```python
from build123d import *

# Parameters (mm, degrees)
F1_DEPTH = 18


with BuildPart() as f1:
    # F0 (on Front) → F1 (new body)
    with BuildSketch(Plane.XZ):
        with BuildLine():
            Line((295, -217), (-317, -217))
            add(Edge.make_bspline(
                [(167, -341), (73.2052326202, -351.3030406237), (-82.9134855426, -352.2458970512), (-215.8919105735, -315.6215987583), (-316.2735343339, -258.65300402), (-317, -217)],
                knots=[0, 0, 0, 0, 0.4043982891, 0.7107448428, 1, 1, 1, 1], degree=3))
            Line((167, -341), (167, -329))
            Line((167, -329), (295, -329))
            Line((295, -329), (295, -217))
        make_face()
        with BuildLine():
            add(Edge.make_bspline(
                [(167, -93), (73.2052326202, -82.6969593763), (-82.9134855426, -81.7541029488), (-215.8919105735, -118.3784012417), (-316.2735343339, -175.34699598), (-317, -217)],
                knots=[0, 0, 0, 0, 0.4043982891, 0.7107448428, 1, 1, 1, 1], degree=3))
            Line((-317, -217), (295, -217))
            Line((295, -217), (295, -105))
            Line((295, -105), (167, -105))
            Line((167, -105), (167, -93))
        make_face()
    extrude(amount=F1_DEPTH)


solid = f1.part
```
For this review, take the finished solid that the model builds, in its own axes (mm). A direction names the side the tool comes from. Coordinates: 2 decimals unless noted, no trailing zeros. Loops run counter-clockwise (first coordinate to the right, second up) from the corner with the lowest first, then second, coordinate; pieces in that order, holes last. Notation, with made-up numbers: (64.25, -5) -> (85.25, -5) arc R24 cw to (85.25, 19) -> close; hole circle Ø10 at (33, 32). An arc over 180 degrees is marked (long way). Return JSON: item names as keys, results as strings. Group by question number.
(1) To check wall thickness, follow L1, parallel to Z at x = 214, y = -11; L2, parallel to Z at x = 15.5, y = -13.5; L3, parallel to X at y = -2, z = -184.5. State the ranges of each line that lie inside material, in increasing order.
(2) Consider section A-A, the plane x = 174. Give the boundary of the cut face in (y, z).
(3) For pin 1 Ø9.5 at (y, z) = (-10.5, -96.5) entering from +X; pin 2 Ø10 at (y, z) = (-5.5, -275) entering from -X; pin 3 Ø2 at (x, y) = (-4, -3.5) entering from +Z, all flat-tipped, find the tip position at first contact; note any pin that passes through.
(4) Tool access review of faces 1 (the flat face through (-15, -18, -215)), 2 (the flat face through (232, -9, -105)), 3 (the flat face through (167, -9, -335)): name each direction out of +Z, -Z, +X, -X, +Y, -Y from which nothing blocks a thin tool from reaching the whole face with its end or side.
Results below:
{
 "1": {"L1": "z = -329 to -105", "L2": "z = -349.3 to -84.7", "L3": "x = -305.79 to 295"},
 "2": {"outline": "(-18, -329) -> (0, -329) -> (0, -105) -> (-18, -105) -> close"},
 "3": {"pin 1": "stops at x = 167", "pin 2": "stops at x = -286.15", "pin 3": "stops at z = -84.95"},
 "4": {"face 1": "+Z, -Z, +X, -X, -Y", "face 2": "+Z, +X, +Y, -Y", "face 3": "-Z, +X, +Y, -Y"}
}
